Check sheet for the drawn part. Datum: minimum x, y, z corner. Units: mm. Give positions to 0.01 mm unless a question says otherwise; leave off trailing zeros. Write each loop counter-clockwise with the first axis right and the second up, starting at its lowest first coordinate (ties: lowest second). Pieces come first, ordered by that corner, then holes. Notation, with made-up numbers: M 65.25,20.5 L 87.25,20.5 A23 cw 87.25,36.5 Z; hole C 18,20.5 d7. An arc over 180 degrees is marked long. Write item = value, one per line. Start each with the question number.
1) Sectioned sample at D-D, the plane y = 6. Count the separate pieces of the cut face and the enclosed holes in it, then the cut area to 3 significant figures.
2) Sectioned sample at C-C, the plane x = 645. Record the cut outline in (y, z) (3 decimals), then the cut area to 3 significant figures.
3) Scan lines: L1, parallel to Z at x = 359.5, y = 11.5 (3 decimals); L2, parallel to Z at x = 662.5, y = 18.25 (3 decimals); L3, parallel to X at y = 15, z = 183. Record each from-to range of solid material in increasing order.
4) Sectioned sample at B-B, the plane z = 474. Record the cut outline in (x, y), then the cut area to 3 significant figures.
5) Sectioned sample at A-A, the plane x = 226. Record the cut outline in (y, z) (3 decimals).
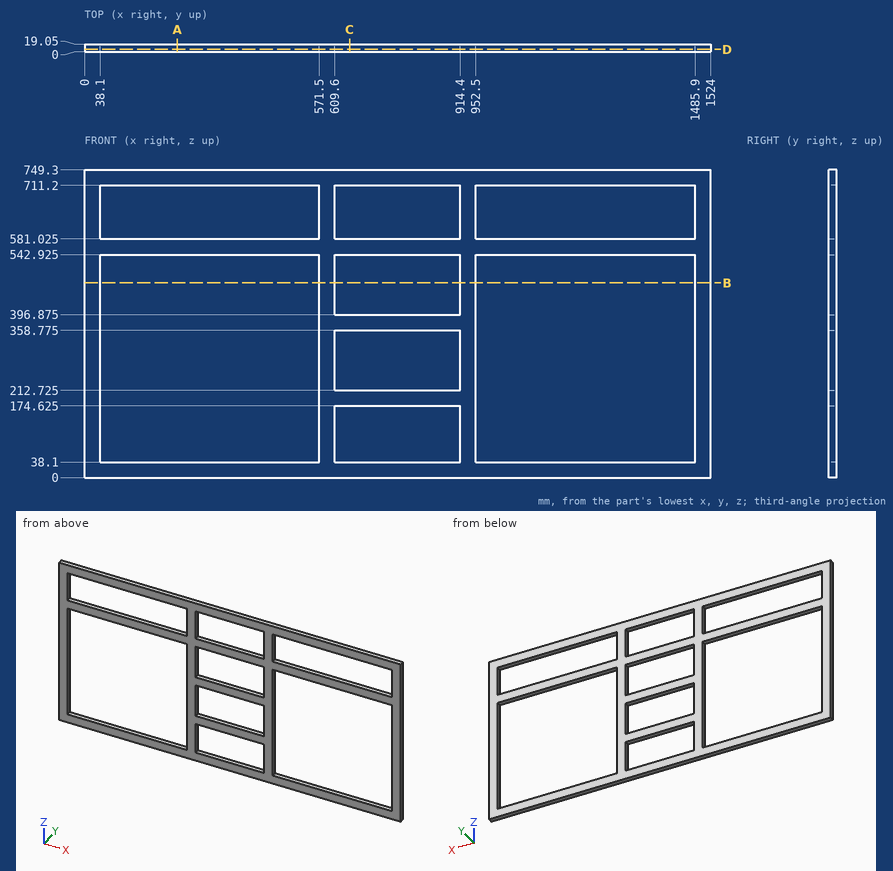
Data:
q1.separate_pieces = 1
q1.enclosed_holes = 8
q1.area = 294,000 mm2
q2.outline = M 0,0 L 19.05,0 L 19.05,38.1 L 0,38.1 Z; M 0,174.625 L 19.05,174.625 L 19.05,212.725 L 0,212.725 Z; M 0,358.775 L 19.05,358.775 L 19.05,396.875 L 0,396.875 Z; M 0,542.925 L 19.05,542.925 L 19.05,581.025 L 0,581.025 Z; M 0,711.2 L 19.05,711.2 L 19.05,749.3 L 0,749.3 Z
q2.area = 3,630 mm2
q3.L1 = 0 to 38.1, 542.925 to 581.025, 711.2 to 749.3
q3.L2 = 0 to 38.1, 174.625 to 212.725, 358.775 to 396.875, 542.925 to 581.025, 711.2 to 749.3
q3.L3 = 0 to 38.1, 571.5 to 952.5, 1485.9 to 1524
q4.outline = M 0,0 L 38.1,0 L 38.1,19.05 L 0,19.05 Z; M 571.5,0 L 609.6,0 L 609.6,19.05 L 571.5,19.05 Z; M 914.4,0 L 952.5,0 L 952.5,19.05 L 914.4,19.05 Z; M 1485.9,0 L 1524,0 L 1524,19.05 L 1485.9,19.05 Z
q4.area = 2,900 mm2
q5.outline = M 0,0 L 19.05,0 L 19.05,38.1 L 0,38.1 Z; M 0,542.925 L 19.05,542.925 L 19.05,581.025 L 0,581.025 Z; M 0,711.2 L 19.05,711.2 L 19.05,749.3 L 0,749.3 Z
